```python
from build123d import *

# Parameters (mm, degrees)
BOSS_EXTRUDE1_DEPTH = 7
SKETCH5_R           = 1.799999865
SKETCH5_R_2         = 1.8
CUT_EXTRUDE4_DEPTH  = 18.482133737
SKETCH2_W           = 6.5
SKETCH2_H           = 1.8
CUT_EXTRUDE1_DEPTH  = 0.5
CUT_EXTRUDE5_DEPTH  = 2.5
CHAMFER1_SIZE       = 1.25
CHAMFER1_SIZE2      = 1.785185008
FILLET1_R           = 3
BOSS_EXTRUDE2_START = -0.6
SKETCH7_R           = 1.799999865
SKETCH7_R_2         = 1.8
BOSS_EXTRUDE2_DEPTH = 0.6
SKETCH8_R           = 1.399999865
SKETCH8_R_2         = 0.599999865
SKETCH8_R_3         = 1.4
SKETCH8_R_4         = 0.6
BOSS_EXTRUDE3_DEPTH = 2.5


with BuildPart() as part:
    # Sketch1 → Boss-Extrude1 (new body)
    with BuildSketch(Plane.XY):
        with BuildLine():
            ThreePointArc((6.631560259, -5.739560401), (3.2, -5), (-0.231560259, -5.739560401))
            ThreePointArc((-0.231560259, -5.739560401), (-8.35, -0.5), (-0.231560259, 4.739560401))
            ThreePointArc((-0.231560259, 4.739560401), (3.2, 4), (6.631560259, 4.739560401))
            ThreePointArc((6.631560259, 4.739560401), (14.75, -0.5), (6.631560259, -5.739560401))
        make_face()
    extrude(amount=-BOSS_EXTRUDE1_DEPTH)

    # Sketch5 → Cut-Extrude4 (cut, through all)
    with BuildSketch(Plane.XY):
        with Locations((9, -0.5)):
            Circle(SKETCH5_R)
        with Locations((-2.6, -0.5)):
            Circle(SKETCH5_R_2)
    extrude(amount=-CUT_EXTRUDE4_DEPTH, mode=Mode.SUBTRACT)

    # Sketch2 → Cut-Extrude1 (cut)
    with BuildSketch(Plane.XY):
        with Locations((3.200000135, 2)):
            Rectangle(SKETCH2_W, SKETCH2_H)
        with Locations((3.200000135, -0.5)):
            Rectangle(SKETCH2_W, SKETCH2_H)
        with BuildLine():
            Line((6.450000135, -4.6), (-0.049999865, -4.6))
            Line((-0.049999865, -4.6), (-0.049999865, -5.660076856))
            ThreePointArc((-0.049999865, -5.660076856), (3.200000146, -5), (6.450000135, -5.660076971))
            Line((6.450000135, -5.660076971), (6.450000135, -4.6))
        make_face()
        with Locations((3.200000135, -3)):
            Rectangle(SKETCH2_W, SKETCH2_H)
        with BuildLine():
            Line((6.450000135, 3.6), (6.450000135, 4.660076971))
            ThreePointArc((6.450000135, 4.660076971), (3.200000146, 4), (-0.049999865, 4.660076856))
            Line((-0.049999865, 4.660076856), (-0.049999865, 3.6))
            Line((-0.049999865, 3.6), (6.450000135, 3.6))
        make_face()
    extrude(amount=-CUT_EXTRUDE1_DEPTH, mode=Mode.SUBTRACT)

    # Sketch6 → Cut-Extrude5 (cut)
    with BuildSketch(Plane(origin=(0, 0, -7), x_dir=(-1, 0, 0), z_dir=(0, 0, -1))):
        Polygon((-0.979571669, -0.5), (0.810214166, -3.6), (4.389785834, -3.6), (6.179571669, -0.5), (4.389785834, 2.6), (0.810214166, 2.6), align=None)
        Polygon((-5.420428331, -0.5), (-7.210214166, 2.6), (-10.789785834, 2.6), (-12.579571669, -0.5), (-10.789785834, -3.6), (-7.210214166, -3.6), align=None)
    extrude(amount=-CUT_EXTRUDE5_DEPTH, mode=Mode.SUBTRACT)

    # Chamfer1
    chamfer1_edges = [part.edges().sort_by_distance(p)[0] for p in [
        (-8.35, -0.5, -7),
        (3.2, -5, -7),
        (14.75, -0.5, -7),
        (3.2, 4, -7),
    ]]
    chamfer1_side = [part.faces().sort_by_distance(p)[0] for p in [
        (3.2, -0.5, -7),
    ]]
    chamfer(chamfer1_edges, length=CHAMFER1_SIZE, length2=CHAMFER1_SIZE2, reference=chamfer1_side[0])

    # Fillet1
    # the kernel refuses this fillet: 3 mm, written as the material it takes off along each edge
    with BuildSketch(Plane(origin=(9, -0.5, -5.214814992), x_dir=(-0.41190256373837064, 0.9112278957460408, 0), z_dir=(-0.9112278957460408, -0.41190256373837064, 0))) as fillet1_piece_1:
        with BuildLine():
            CenterArc((5.75 - FILLET1_R, -FILLET1_R * 0.315298788879), FILLET1_R, 0, 35)
            Line((5.75 - FILLET1_R * 0.180847955711, FILLET1_R * 0.258277647472), (5.75, 0))
            Line((5.75, 0), (5.75, -FILLET1_R * 0.315298788879))
        make_face()
    fillet1_piece_1_solid = revolve(axis=Axis((9, -0.5, -5.214814992), (0, 0, -1)), revolution_arc=228.648814079, mode=Mode.PRIVATE)
    with BuildSketch(Plane(origin=(3.2, 12.331, -5.214814992), x_dir=(-0.41190256373837086, -0.9112278957460408, 0), z_dir=(-0.9112278957460408, 0.41190256373837086, 0))) as fillet1_piece_2:
        with BuildLine():
            CenterArc((8.331 + FILLET1_R, FILLET1_R * 0.315298788879), FILLET1_R, 180, 35)
            Line((8.331 + FILLET1_R * 0.180847955711, -FILLET1_R * 0.258277647472), (8.331, 0))
            Line((8.331, 0), (8.331, FILLET1_R * 0.315298788879))
        make_face()
    fillet1_piece_2_solid = revolve(axis=Axis((3.2, 12.331, -5.214814992), (0, 0, 1)), revolution_arc=48.648814079, mode=Mode.PRIVATE)
    with BuildSketch(Plane(origin=(3.2, -13.331, -5.214814992), x_dir=(0.41190256373837153, 0.9112278957460405, 0), z_dir=(0.9112278957460405, -0.41190256373837153, 0))) as fillet1_piece_3:
        with BuildLine():
            CenterArc((8.331 + FILLET1_R, FILLET1_R * 0.315298788879), FILLET1_R, 180, 35)
            Line((8.331 + FILLET1_R * 0.180847955711, -FILLET1_R * 0.258277647472), (8.331, 0))
            Line((8.331, 0), (8.331, FILLET1_R * 0.315298788879))
        make_face()
    fillet1_piece_3_solid = revolve(axis=Axis((3.2, -13.331, -5.214814992), (0, 0, 1)), revolution_arc=48.648814079, mode=Mode.PRIVATE)
    with BuildSketch(Plane(origin=(-2.6, -0.5, -5.214814992), x_dir=(0.41190256373837075, -0.9112278957460408, 0), z_dir=(0.9112278957460408, 0.41190256373837075, 0))) as fillet1_piece_4:
        with BuildLine():
            CenterArc((5.75 - FILLET1_R, -FILLET1_R * 0.315298788879), FILLET1_R, 0, 35)
            Line((5.75 - FILLET1_R * 0.180847955711, FILLET1_R * 0.258277647472), (5.75, 0))
            Line((5.75, 0), (5.75, -FILLET1_R * 0.315298788879))
        make_face()
    fillet1_piece_4_solid = revolve(axis=Axis((-2.6, -0.5, -5.214814992), (0, 0, -1)), revolution_arc=228.648814079, mode=Mode.PRIVATE)
    add([fillet1_piece_1_solid, fillet1_piece_2_solid, fillet1_piece_3_solid, fillet1_piece_4_solid], mode=Mode.SUBTRACT)

    # Sketch7 → Boss-Extrude2 (add)
    with BuildSketch(Plane(origin=(0, 0, -4.5), x_dir=(-1, 0, 0), z_dir=(0, 0, -1)).offset(BOSS_EXTRUDE2_START)):
        with Locations(Location((-9, -0.5, 0), (0, 0, 180))):
            Circle(SKETCH7_R)
        with Locations(Location((2.6, -0.5, 0), (0, 0, 180))):
            Circle(SKETCH7_R_2)
    extrude(amount=BOSS_EXTRUDE2_DEPTH)

    # Sketch8 → Boss-Extrude3 (add)
    # profile 1 of 2: a face of its own
    with BuildSketch(Plane(origin=(0, 0, -4.5), x_dir=(-1, 0, 0), z_dir=(0, 0, -1))):
        with Locations(Location((-9, -0.5, 0), (0, 0, 180))):
            Circle(SKETCH8_R)
        with Locations(Location((-9, -0.5, 0), (0, 0, 180))):
            Circle(SKETCH8_R_2, mode=Mode.SUBTRACT)
    # profile 2 of 2: a face of its own
    with BuildSketch(Plane(origin=(0, 0, -4.5), x_dir=(-1, 0, 0), z_dir=(0, 0, -1))):
        with Locations(Location((2.6, -0.5, 0), (0, 0, 180))):
            Circle(SKETCH8_R_3)
        with Locations(Location((2.6, -0.5, 0), (0, 0, 180))):
            Circle(SKETCH8_R_4, mode=Mode.SUBTRACT)
    extrude(amount=BOSS_EXTRUDE3_DEPTH)


solid = part.part
```
The listing builds one solid part. Answer for the finished solid, in the listing's coordinates (mm). A direction names the side the tool comes from. Give positions to 0.01 mm unless a question says otherwise; leave off trailing zeros. Write each loop counter-clockwise with the first axis right and the second up, starting at its lowest first coordinate (ties: lowest second). Pieces come first, ordered by that corner, then holes. Notation, with made-up numbers: (33, 85) -> (81, 85) arc R13 ccw to (81, 104) -> close; hole circle Ø3 at (14, -13.75). An arc over 180 degrees is marked (long way). Write item = value, one per line. Start each with the question number.
1) Which of the six approach directions +Z, -Z, +X, -X, +Y, -Y give full straight-line access (tool end or side, diameter ignored) to faces 5 (the face through (3.2, -4.8, -0.5)), 6 (the face through (3.2, 3.8, -0.5)), 7 (the face through (10.717, 0.041, -1.923)), 8 (the face through (-3, 2.6, -6))?
2) Straight lines are drawn through the part: line 1 along X through (y, z) = (-0.5, -2.8); line 2 along X through (y, z) = (1.75, -6); line 3 along Y through (x, z) = (9, -1.9). For each, find the intervals that lie inside material, in ascending order.
3) The part is cut by section A-A, the plane z = -0.25. Determine the outline of the cut face in (x, y), and give its area (3 significant figures).
4) Determine the mould class of faces 1 (the face through (10, -1, -7)), 2 (the face through (-3, -1, -3.9)), 3 (the face through (3.2, 4, -2.1)), 4 (the face through (14.748, -0.339, -2.105)) for opening direction Y: +Y half, -Y half, draft (parallel to the pull), parting line (faces both ways), or undercut.
5) The part is cut by section B-B, the plane z = -2.5. Determine the outline of the cut face in (x, y).
6) The part is cut by section C-C, the plane z = -5. Count the separate pieces of the cut face and the enclosed holes in it, and give its area (3 significant figures).
7) Each of these flat-tipped pins is pushed along its axis until it touches: pin 1 (3 mm diameter, centred on x = -2.5, z = -6, fed in from +Y); pin 2 (1 mm diameter, centred on y = -2.5, z = -5.5, fed in from +X); pin 3 (0.6 mm diameter, centred on x = 2, z = -0.5, fed in from -Y); pin 4 (0.5 mm diameter, centred on x = 3, y = -5.5, fed in from +Z). Where does it stop, or does it pass through?
Solutions:
q1.face_5 = +Z, -Y
q1.face_6 = +Z, +Y
q1.face_7 = +Z
q1.face_8 = -Z
q2.line_1 = -8.35 to -4.4, -0.8 to 7.2, 10.8 to 14.75
q2.line_2 = -7.29 to -4.88, -0.32 to 6.72, 11.28 to 13.69
q2.line_3 = -6.25 to -2.3, 1.3 to 5.25
q3.outline = (-0.23, -5.74) arc R8.33 cw to (-0.05, -5.66) -> (-0.05, -4.6) -> (6.45, -4.6) -> (6.45, -5.66) arc R8.33 cw to (6.63, -5.74) arc R5.75 ccw (long way) to (6.63, 4.74) arc R8.33 cw to (6.45, 4.66) -> (6.45, 3.6) -> (-0.05, 3.6) -> (-0.05, 4.66) arc R8.33 cw to (-0.23, 4.74) arc R5.75 ccw (long way) to start; hole circle Ø3.6 at (-2.6, -0.5); hole (-0.05, -3.9) -> (6.45, -3.9) -> (6.45, -2.1) -> (-0.05, -2.1) -> close; hole (-0.05, -1.4) -> (6.45, -1.4) -> (6.45, 0.4) -> (-0.05, 0.4) -> close; hole (-0.05, 1.1) -> (6.45, 1.1) -> (6.45, 2.9) -> (-0.05, 2.9) -> close; hole circle Ø3.6 at (9, -0.5)
q3.area = 158 mm²
q4.face_1 = draft
q4.face_2 = undercut
q4.face_3 = +Y half
q4.face_4 = parting line
q5.outline = (-0.23, -5.74) arc R8.33 cw to (6.63, -5.74) arc R5.75 ccw (long way) to (6.63, 4.74) arc R8.33 cw to (-0.23, 4.74) arc R5.75 ccw (long way) to start; hole circle Ø3.6 at (-2.6, -0.5); hole circle Ø3.6 at (9, -0.5)
q6.separate_pieces = 3
q6.enclosed_holes = 4
q6.area = 160 mm²
q7.pin_1 = 5.24
q7.pin_2 = 14.37
q7.pin_3 = -5.14
q7.pin_4 = through
